from build123d import *

# Parameters (mm, degrees)
F0_W     = 527.05
F0_H     = 76.2
F1_DEPTH = 6.35
F2_W     = 6.35
F2_H     = 6.35
F2_W_2   = 25.4
F2_H_2   = 12.7
F2_H_3   = 25.4
F3_DEPTH = 6.35
F4_W     = 6.35
F4_H     = 12.7
F5_DEPTH = 25.4


with BuildPart() as f1:
    # F0 (on Right) → F1 (new body)
    with BuildSketch(Plane.YZ):
        Rectangle(F0_W, F0_H)
    extrude(amount=F1_DEPTH)

    # F2 (on face) → F3 (cut, through all)
    with BuildSketch(Plane.YZ.offset(6.35)):
        Polygon((-263.525, -31.75), (-263.525, -38.1), (-238.125, -38.1), (-238.125, -31.75), (-257.175, -31.75), align=None)
        with Locations((-260.35, -28.575)):
            Rectangle(F2_W, F2_H)
        with Locations((-200.66, -34.925)):
            Rectangle(F2_W_2, F2_H)
        with Locations((-150.495, -34.925)):
            Rectangle(F2_W_2, F2_H)
        with Locations((-100.33, -34.925)):
            Rectangle(F2_W_2, F2_H)
        with Locations((-50.165, -34.925)):
            Rectangle(F2_W_2, F2_H)
        with Locations((0, -34.925)):
            Rectangle(F2_W_2, F2_H)
        with Locations((50.165, -34.925)):
            Rectangle(F2_W_2, F2_H)
        with Locations((100.33, -34.925)):
            Rectangle(F2_W_2, F2_H)
        with Locations((150.495, -34.925)):
            Rectangle(F2_W_2, F2_H)
        with Locations((200.66, -34.925)):
            Rectangle(F2_W_2, F2_H)
        Polygon((238.125, -31.75), (238.125, -38.1), (263.525, -38.1), (263.525, -31.75), (257.175, -31.75), align=None)
        with Locations((260.35, -28.575)):
            Rectangle(F2_W, F2_H)
        with Locations((-260.35, 31.75)):
            Rectangle(F2_W, F2_H_2)
        with Locations((-260.35, 0)):
            Rectangle(F2_W, F2_H_3)
        with Locations((260.35, 31.75)):
            Rectangle(F2_W, F2_H_2)
        with Locations((260.35, 0)):
            Rectangle(F2_W, F2_H_3)
    extrude(amount=-F3_DEPTH, mode=Mode.SUBTRACT)

    # F4 (on face) → F5 (cut)
    with BuildSketch(Plane.YZ.offset(6.35)):
        with Locations((177.8, 19.05)):
            Rectangle(F4_W, F4_H)
        with Locations((177.8, -25.4)):
            Rectangle(F4_W, F4_H)
    extrude(amount=-F5_DEPTH, mode=Mode.SUBTRACT)


solid = f1.part
The listing builds one solid part. Answer for the finished solid, in the listing's coordinates (mm). Give positions to 0.01 mm unless a question says otherwise; leave off trailing zeros. Write each loop counter-clockwise with the first axis right and the second up, starting at its lowest first coordinate (ties: lowest second). Pieces come first, ordered by that corner, then holes.
1) Section C-C (x = 1.5) is taken. Count the separate pieces of the cut face and the enclosed holes in it, and give its area (3 significant figures).
2) Given P1, Ø1.9, axis at x = 4, z = -34, coming from the -Y side (3 decimals); P2, Ø3, axis at x = 4.5, z = -27, coming from the -Y side (3 decimals); P3, Ø1.9, axis at x = 4.5, z = -28, coming from the +Y side (3 decimals), each flat-ended and moving along its own axis, determine where each tip first touches the part or whether it passes through.
3) Section B-B (y = -2) is taken. Write down the section's boundary in (x, z).
4) Section A-A (z = -3) is taken. Write down the section's boundary in (x, y) (3 decimals), and give its area (3 significant figures).
5) Find the intervals of material crossed by L1, parallel to Y at x = 6, z = -31 (3 decimals); L2, parallel to Y at x = 5.75, z = 22.5 (3 decimals); L3, parallel to Z at x = 0.75, y = -39.5, in increasing order.
Response:
1. separate pieces: 1
1. enclosed holes: 2
1. area: 37,700 mm2
2. P1: stops at y = -238.125
2. P2: stops at y = -257.175
2. P3: stops at y = 257.175
3. outline: (0, -31.75) - (6.35, -31.75) - (6.35, 38.1) - (0, 38.1) - close
4. outline: (0, -257.175) - (6.35, -257.175) - (6.35, 257.175) - (0, 257.175) - close
4. area: 3,270 mm2
5. L1: y = -257.175 to 174.625, 180.975 to 257.175
5. L2: y = -263.525 to 174.625, 180.975 to 263.525
5. L3: z = -31.75 to 38.1
